Read the model definition and answer for the solid it produces. Units are mm, in the model's axes. Face numbers are marked on the shaded views. A direction names the side the tool comes from. Give positions to 0.01 mm unless a question says otherwise; leave off trailing zeros. Loops run counter-clockwise (first coordinate to the right, second up) from the corner with the lowest first, then second, coordinate; pieces in that order, holes last. Notation, with made-up numbers: (86, 47.5) - (130, 47.5) arc R15 ccw to (130, 66.5) - close; hole circle Ø4 at (-26.5, -13.5). An arc over 180 degrees is marked (long way). Put each result on its own line as item: value. Start each with the question number.
1. Consider L1, parallel to X at y = 8.75, z = 27.94; L2, parallel to Y at x = 10.7, z = 27.94; L3, parallel to Y at x = 9.9, z = 27.94. Determine where each line is inside the solid, lowest interval first. Write a range as from..to.
2. For the marked faces 1, 2 and 3, determine the directions among +Z, -Z, +X, -X, +Y, -Y from which every point of the face is accessible in a straight line to the end or side of a thin tool.
3. A cutting plane is placed at A-A, the plane y = 0. Determine the outline of the cut face in (x, z), plus the area to 3 significant figures.
4. A cutting plane is placed at C-C, the plane z = 22.5. Determine the outline of the cut face in (x, y) (1 decimal).
5. A cutting plane is placed at D-D, the plane z = 27.94. Count the separate pieces of the cut face and the enclosed holes in it, plus the area to 3 significant figures.
6. For a pull along X with two mould halves and no side action, classify the marked faces 4, 5, 6 and 7 as released by +X, released by -X, zero draft, split by the parting line, or undercut.
7. Given pin 1 Ø3 at (y, z) = (-28, 27.5) entering from -X; pin 2 Ø16 at (x, y) = (-15, 14) entering from -Z; pin 3 Ø1 at (y, z) = (23, 26) entering from +X; pin 4 Ø8 at (y, z) = (25, 6.5) entering from -X, each flat-ended and moving along its own axis, determine where each tip first touches the part or whether it passes through.
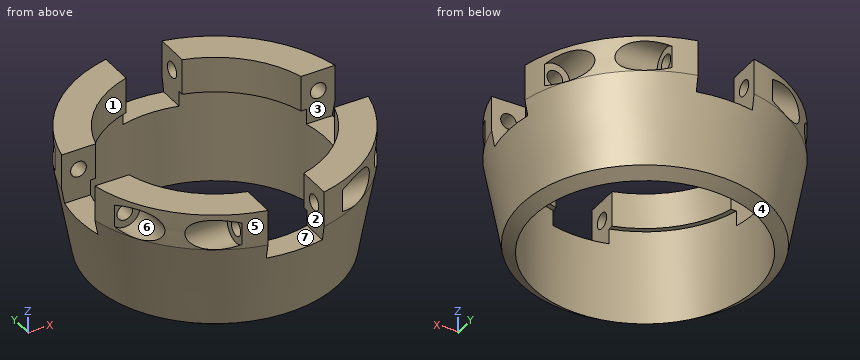
```python
from build123d import *

# Parameters (mm, degrees)
PULLEY_RECESS_START = -12.7
SKETCH5_W           = 13.97
SKETCH5_H           = 12.7
PULLEY_RECESS_DEPTH = 72.92587845
CIRPATTERN1_COUNT   = 4
CHAMFER1_SIZE       = 2.54
CHAMFER1_SIZE_2     = 3.165934508


with BuildPart() as part:
    # Sketch1 → base_ring (revolve)
    with BuildSketch(Plane.YZ, mode=Mode.PRIVATE) as base_ring_sk:
        Polygon((27.78125, 0), (27.78125, 24.13), (26.51125, 24.13), (26.51125, 33.02), (34.76625, 33.02), (34.76625, 24.13), (30.32125, 0), align=None)
    revolve(base_ring_sk.sketch.rotate(Axis((0, 0, 0), (0, 0, 1)), 90), axis=Axis((0, 0, 0), (0, 0, 1)))

    # Sketch5 → pulley_recess (cut)
    with BuildSketch(Plane.XY.offset(33.02).offset(PULLEY_RECESS_START)):
        with Locations((0, 31.924521531)):
            Rectangle(SKETCH5_W, SKETCH5_H)
    pulley_recess = extrude(amount=PULLEY_RECESS_DEPTH, mode=Mode.SUBTRACT)

    # Sketch8 → pulley_bolt_hole (revolve, cut)
    with BuildSketch(Plane(origin=(34.76625, 29.86633275, 27.94), x_dir=(0, 0, -1), z_dir=(0, 1, 0))):
        Polygon((0, 0), (0, 39.275163199), (1.9558, 38.1), (1.9558, 22.3012), (3.77063, 22.3012), (3.77063, 0), align=None)
    pulley_bolt_hole = revolve(axis=Axis((41.11625, 29.86633275, 27.94), (-1, 0, 0)), mode=Mode.SUBTRACT)

    # bolthole_mirror: pulley_bolt_hole across plane
    add(pulley_bolt_hole.mirror(Plane(origin=(0, 0, 0), x_dir=(0, 0, 1), z_dir=(1, 0, 0))), mode=Mode.SUBTRACT)

    # CirPattern1: pulley_recess, pulley_bolt_hole ×4 about axis
    cirpattern1_axis = Axis((0, 0, 0), (0, 0, 1))
    add([pulley_recess.rotate(cirpattern1_axis, i * 360 / CIRPATTERN1_COUNT) for i in range(1, CIRPATTERN1_COUNT)], mode=Mode.SUBTRACT)
    add([pulley_bolt_hole.rotate(cirpattern1_axis, i * 360 / CIRPATTERN1_COUNT) for i in range(1, CIRPATTERN1_COUNT)], mode=Mode.SUBTRACT)

    # CirPattern1 copy 1 sketch → CirPattern1 copy 1 (revolve, cut)
    with BuildSketch(Plane(origin=(-29.86633275, -34.76625, 27.94), x_dir=(0, 0, -1), z_dir=(-1, 0, 0))):
        Polygon((0, 0), (0, -39.275163199), (1.9558, -38.1), (1.9558, -22.3012), (3.77063, -22.3012), (3.77063, 0), align=None)
    revolve(axis=Axis((-29.86633275, -41.11625, 27.94), (0, -1, 0)), mode=Mode.SUBTRACT)

    # CirPattern1 copy 2 sketch → CirPattern1 copy 2 (revolve, cut)
    with BuildSketch(Plane(origin=(34.76625, -29.86633275, 27.94), x_dir=(0, 0, -1), z_dir=(0, -1, 0))):
        Polygon((0, 0), (0, -39.275163199), (1.9558, -38.1), (1.9558, -22.3012), (3.77063, -22.3012), (3.77063, 0), align=None)
    revolve(axis=Axis((41.11625, -29.86633275, 27.94), (1, 0, 0)), mode=Mode.SUBTRACT)

    # CirPattern1 copy 3 sketch → CirPattern1 copy 3 (revolve, cut)
    with BuildSketch(Plane(origin=(29.86633275, 34.76625, 27.94), x_dir=(0, 0, -1), z_dir=(1, 0, 0))):
        Polygon((0, 0), (0, -39.275163199), (1.9558, -38.1), (1.9558, -22.3012), (3.77063, -22.3012), (3.77063, 0), align=None)
    revolve(axis=Axis((29.86633275, 41.11625, 27.94), (0, 1, 0)), mode=Mode.SUBTRACT)

    # Chamfer1
    # the kernel refuses this chamfer: 3.165934508, 2.54 mm, written as the material it takes off along each edge
    with BuildSketch(Plane(origin=(0, 0, 0), x_dir=(-1, 0, 0), z_dir=(0, 1, 0))) as chamfer1_piece_1:
        Polygon((30.32125 + CHAMFER1_SIZE * 0.181162429477, CHAMFER1_SIZE * 0.983453188589), (30.32125 - CHAMFER1_SIZE_2, 0), (30.32125, 0), align=None)
    revolve(axis=Axis((0, 0, 0), (0, 0, 1)), mode=Mode.SUBTRACT)


solid = part.part
```
Return value:
1. L1: x = -33.65..-31.82, -27.91..-25.03, 25.03..27.91, 31.82..33.65
1. L2: y = -33.08..-31.82, -27.91..-24.26, 24.26..27.91, 31.82..33.08
1. L3: y = -33.33..-31.82, -27.91..-24.59, 24.59..27.91, 31.82..33.33
2. face 1: +Z, -Z
2. face 2: +Z, +Y, -Y
2. face 3: +Z, +X, -X
3. outline: (-34.06, 20.32) - (-30.78, 2.5) - (-27.78, 0.43) - (-27.78, 20.32) - close; (27.78, 0.43) - (30.78, 2.5) - (34.06, 20.32) - (27.78, 20.32) - close
3. area: 172 mm2
4. outline: (-33.8, -7) arc R34.5 ccw to (-7, -33.8) - (-7, -26.9) arc R27.8 cw to (-26.9, -7) - close; (-33.8, 7) - (-26.9, 7) arc R27.8 cw to (-7, 26.9) - (-7, 33.8) arc R34.5 ccw to start; (7, -33.8) arc R34.5 ccw to (33.8, -7) - (26.9, -7) arc R27.8 cw to (7, -26.9) - close; (7, 26.9) arc R27.8 cw to (26.9, 7) - (33.8, 7) arc R34.5 ccw to (7, 33.8) - close
5. separate pieces: 12
5. enclosed holes: 0
5. area: 649 mm2
6. face 4: split by the parting line
6. face 5: released by -X
6. face 6: undercut
6. face 7: undercut
7. pin 1: stops at x = -12.47
7. pin 2: stops at z = 0.43
7. pin 3: stops at x = 26.5
7. pin 4: stops at x = -23.64
